Autodesk Inventor part; units mm, degrees
ref_plane "YZ Plane" through (0, 0, 0) normal (1, 0, 0) x (0, 1, 0)
ref_plane "XZ Plane" through (0, 0, 0) normal (0, 1, 0) x (-1, 0, 0)
ref_plane "XY Plane" through (0, 0, 0) normal (0, 0, 1) x (1, 0, 0)
sketch "Sketch1" plane through (0, 0, 0) normal (0, 1, 0) x (-1, 0, 0)
  circle A0 centre (0, 0) radius 7.6
  circle A1 centre (0, 0) radius 9.7
  dimension "d0" = 15.2
  dimension "d1" = 19.4
extrude "Extrusion1" add sketch "Sketch1" along normal blind 2 contours A0 | A1
extrude "Extrusion2" add sketch "Sketch1" against normal blind 10 contours A0
sketch "Sketch2" plane through (0, 0, 0) normal (1, 0, 0) x (0, 1, 0)
  circle A0 centre (-5, 0) radius 2.25
  line L0 (0, -9.7) -> (0, 9.7)
  point P0 (0, 0)
  dimension "d6" = 4.5
  dimension "d7" = 5
extrude "Extrusion3" cut sketch "Sketch2" along normal blind 23
sketch "Sketch3" plane through (0, -10, 0) normal (0, -1, 0) x (1, 0, 0)
  circle A0 centre (0, 0) radius 3.75
  circle A1 centre (0, 0) radius 5.75
  dimension "d10" = 7.5
  dimension "d11" = 2
extrude "Extrusion4" add sketch "Sketch3" along normal blind 5
sketch "Sketch6" plane through (0, -10, 0) normal (0, -1, 0) x (1, 0, 0)
  circle A0 centre (0, 0) radius 3.75
  circle A1 centre (-1.5, -1.75) radius 1.25
  circle A2 centre (-1.5, 1.75) radius 1.25
  line L0 (-1.5, -3.4369) -> (-1.5, 3.4369) construction
  line L1 (-1.5, -1.75) -> (-1.5, 1.75)
  point P0 (-1.5, 0)
  dimension "d18" = 2.5
  dimension "d24" = 3.5
  dimension "d25" = 1.5
extrude "Extrusion6" cut sketch "Sketch6" against normal up to next contours A1 | A2
properties part number "button bottom plug"
Verification items for the finished model (mm, model axes). A direction names the side the tool comes from. Round coordinates to 2 decimals unless told otherwise and drop trailing zeros. Write each loop counter-clockwise with the first axis right and the second up, starting at its lowest first coordinate (ties: lowest second). Pieces come first, ordered by that corner, then holes.
(1) Mould release check, pull along X, two halves, no side actions. Record for faces 1 (the cylindrical face through (-0.75, -12.46, -5.7)), 2 (the flat face through (1, -10, 6)), 3 (the cylindrical face through (-0.3, -4.1, -1.4)): pulls with the +X half, pulls with the -X half, needs draft (parallel to the pull), parting line crosses it, or undercut.
Returned:
face 1: parting line crosses it
face 2: needs draft
face 3: undercut
(2) Access from +Z, -Z, +X, -X, +Y, -Y to the whole of each face (thin tool, end or side, straight path). Record for faces 4 (the flat face through (6, 0, -5)), 5 (the cylindrical face through (3.748, -2.854, -0.676)), 6 (the cylindrical face through (-9.252, 0.986, -2.914)).
Returned:
face 4: -Y
face 5: +X
face 6: +Y, -Y
(3) Section check B-B (z = -1.75). Enter the section's corners in (x, y).
Returned:
outline: (-9.54, 0) - (-7.4, 0) - (-7.4, -10) - (-5.48, -10) - (-5.48, -15) - (-3.32, -15) - (-3.32, -10) - (-2.75, -10) - (-2.75, 2) - (-9.54, 2) - close; (-0.25, -10) - (3.32, -10) - (3.32, -15) - (5.48, -15) - (5.48, -10) - (7.4, -10) - (7.4, -6.41) - (0, -6.41) - (0, -3.59) - (7.4, -3.59) - (7.4, 0) - (9.54, 0) - (9.54, 2) - (-0.25, 2) - close
(4) Section check C-C (y = -11.25). Enter the section's corners in (x, z).
Returned:
outline: circle Ø11.5 at (0, 0); hole circle Ø7.5 at (0, 0)
(5) Section check A-A (x = -1). Enter the section's corners in (y, z), plus the area to 3 significant figures.
Returned:
outline: (-15, -5.66) - (-10, -5.66) - (-10, -7.53) - (0, -7.53) - (0, -9.65) - (2, -9.65) - (2, -2.9) - (-10, -2.9) - (-10, -3.61) - (-15, -3.61) - close; (-15, 3.61) - (-10, 3.61) - (-10, 2.9) - (2, 2.9) - (2, 9.65) - (0, 9.65) - (0, 7.53) - (-10, 7.53) - (-10, 5.66) - (-15, 5.66) - close; (-10, -0.6) - (2, -0.6) - (2, 0.6) - (-10, 0.6) - close
area: 155 mm2
(6) Material ranges on line 1 (Z direction, x = -1.5, y = -0.75); line 2 (Y direction, x = 5.5, z = -5); line 3 (Y direction, x = 3, z = 1.5), recorded low to high.
Returned:
line 1: z = -7.45 to -3, -0.5 to 0.5, 3 to 7.45
line 2: y = -10 to 2
line 3: y = -10 to -6.68, -3.32 to 2
(7) Section check D-D (x = 5). Enter the section's corners in (y, z), plus the area to 3 significant figures.
Returned:
outline: (-15, -2.84) - (-10, -2.84) - (-10, -5.72) - (0, -5.72) - (0, -8.31) - (2, -8.31) - (2, 8.31) - (0, 8.31) - (0, 5.72) - (-10, 5.72) - (-10, 2.84) - (-15, 2.84) - close; hole circle Ø4.5 at (-5, 0)
area: 160 mm2
(8) Depth check by flat-ended pin: pin 1 Ø6 at (x, z) = (0, 0) entering from -Y; pin 2 Ø3 at (y, z) = (-6, 0) entering from +X; pin 3 Ø1.5 at (x, z) = (-1.5, -1.75) entering from -Y; pin 4 Ø8 at (y, z) = (-6, 5.5) entering from +X. Enter the tip coordinate at first touch or a pass-through.
Returned:
pin 1: stops at y = -10
pin 2: stops at x = 7.6
pin 3: passes through
pin 4: stops at x = 7.44
